Input: part model. Units: mm. Frame: model coordinates. A direction names the side the tool comes from. Coordinates: 2 decimals unless noted, no trailing zeros. Order: outer loops, then holes, each group sorted by start corner. A loop starts at its lowest first (then second) coordinate and runs counter-clockwise, first axis right, second up. Notation, with made-up numbers: (64.25, 32.5) -> (118.25, 32.5) arc R29 ccw to (118.25, 54.5) -> close; hole circle Ø7 at (54.25, 6.25). An arc over 180 degrees is marked (long way). One line per question, with ' | ' between items.
```python
from build123d import *

# Parameters (mm, degrees)
BOX004_W               = 20
BOX004_H               = 20
BOX004_DEPTH           = 80
BOX003_W               = 20
BOX003_H               = 20
BOX003_DEPTH           = 80
BOX002_W               = 10
BOX002_H               = 25
BOX002_DEPTH           = 35
BOX002_PITCH_ANGLE     = -15
BOX001_W               = 10
BOX001_H               = 25
BOX001_DEPTH           = 35
BOX001_PITCH_ANGLE     = 15
BOX_W                  = 20
BOX_H                  = 25
BOX_DEPTH              = 35
CYLINDER005_R          = 10
CYLINDER005_DEPTH      = 180
CYLINDER005_ROLL_ANGLE = 90
CYLINDER004_R          = 54
CYLINDER004_DEPTH      = 100
CYLINDER003_R          = 59
CYLINDER003_DEPTH      = 10
CYLINDER002_R          = 64
CYLINDER002_DEPTH      = 85
CYLINDER001_R          = 70
CYLINDER001_DEPTH      = 90
CYLINDER_R             = 77.5
CYLINDER_DEPTH         = 10
FILLET_R               = 3
FILLET001_R            = 5
FILLET002_R            = 5


with BuildPart() as tab_cut_l:
    # Box004 → Box004 (new body)
    with BuildSketch(Plane(origin=(-83, -10, 20), x_dir=(1, 0, 0), z_dir=(0, 0, 1))):
        with Locations((10, 10)):
            Rectangle(BOX004_W, BOX004_H)
    extrude(amount=BOX004_DEPTH)


with BuildPart() as tab_cut_r:
    # Box003 → Box003 (new body)
    with BuildSketch(Plane(origin=(63, -10, 20), x_dir=(1, 0, 0), z_dir=(0, 0, 1))):
        with Locations((10, 10)):
            Rectangle(BOX003_W, BOX003_H)
    extrude(amount=BOX003_DEPTH)


with BuildPart() as cube001:
    # Box002 → Box002 (new body)
    with BuildSketch(Plane.XY):
        with Locations((5, 12.5)):
            Rectangle(BOX002_W, BOX002_H)
    extrude(amount=BOX002_DEPTH)


with BuildPart() as cube001_1:
    # Box002 pitch: moved
    add(cube001.part.rotate(Axis((0, 0, 0), (0, 1, 0)), BOX002_PITCH_ANGLE))


with BuildPart() as cube001_2:
    # Box002 placement: moved
    add(cube001_1.part.moved(Location((-9.95, 48, 64))))


with BuildPart() as cube:
    # Box001 → Box001 (new body)
    with BuildSketch(Plane.XY):
        with Locations((5, 12.5)):
            Rectangle(BOX001_W, BOX001_H)
    extrude(amount=BOX001_DEPTH)


with BuildPart() as cube_1:
    # Box001 pitch: moved
    add(cube.part.rotate(Axis((0, 0, 0), (0, 1, 0)), BOX001_PITCH_ANGLE))


with BuildPart() as cube_2:
    # Box001 placement: moved
    add(cube_1.part.moved(Location((0, 48, 65))))


with BuildPart() as bearing_slot:
    # Box → Box (new body)
    with BuildSketch(Plane(origin=(-10, 48, 65), x_dir=(1, 0, 0), z_dir=(0, 0, 1))):
        with Locations((10, 12.5)):
            Rectangle(BOX_W, BOX_H)
    extrude(amount=BOX_DEPTH)


with BuildPart() as bearing_holes:
    # Cylinder005 → Cylinder005 (new body)
    with BuildSketch(Plane.XY):
        Circle(CYLINDER005_R)
    extrude(amount=CYLINDER005_DEPTH)


with BuildPart() as bearing_holes_1:
    # Cylinder005 roll: moved
    add(bearing_holes.part.rotate(Axis((0, 0, 0), (1, 0, 0)), CYLINDER005_ROLL_ANGLE))


with BuildPart() as bearing_holes_2:
    # Cylinder005 placement: moved
    add(bearing_holes_1.part.moved(Location((0, 90, 65))))


with BuildPart() as through_hole:
    # Cylinder004 → Cylinder004 (new body)
    with BuildSketch(Plane.XY):
        Circle(CYLINDER004_R)
    extrude(amount=CYLINDER004_DEPTH)


with BuildPart() as inner_lip:
    # Cylinder003 → Cylinder003 (new body)
    with BuildSketch(Plane.XY.offset(80)):
        Circle(CYLINDER003_R)
    extrude(amount=CYLINDER003_DEPTH)


with BuildPart() as inner_hole:
    # Cylinder002 → Cylinder002 (new body)
    with BuildSketch(Plane.XY):
        Circle(CYLINDER002_R)
    extrude(amount=CYLINDER002_DEPTH)


with BuildPart() as body_cylinder:
    # Cylinder001 → Cylinder001 (new body)
    with BuildSketch(Plane.XY.offset(5)):
        Circle(CYLINDER001_R)
    extrude(amount=CYLINDER001_DEPTH)


with BuildPart() as cut007:
    # Cylinder → Cylinder (new body)
    with BuildSketch(Plane.XY):
        Circle(CYLINDER_R)
    extrude(amount=CYLINDER_DEPTH)

    # Fusion: union Body_Cylinder
    add(body_cylinder.part)

    # Cut: cut Inner_Hole
    add(inner_hole.part, mode=Mode.SUBTRACT)

    # Fusion001: union Inner_Lip
    add(inner_lip.part)

    # Cut001: cut Through_Hole
    add(through_hole.part, mode=Mode.SUBTRACT)

    # Fillet
    fillet_edges = [cut007.edges().sort_by_distance(p)[0] for p in [
        (-70, 0, 10),
    ]]
    fillet(fillet_edges, radius=FILLET_R)

    # Fillet001
    fillet001_edges = [cut007.edges().sort_by_distance(p)[0] for p in [
        (-77.5, 0, 0),
    ]]
    fillet(fillet001_edges, radius=FILLET001_R)

    # Fillet002
    fillet002_edges = [cut007.edges().sort_by_distance(p)[0] for p in [
        (-70, 0, 95),
    ]]
    fillet(fillet002_edges, radius=FILLET002_R)

    # Cut002: cut Bearing_Holes
    add(bearing_holes_2.part, mode=Mode.SUBTRACT)

    # Cut003: cut Bearing_Slot
    add(bearing_slot.part, mode=Mode.SUBTRACT)

    # Cut004: cut Cube
    add(cube_2.part, mode=Mode.SUBTRACT)

    # Cut005: cut Cube001
    add(cube001_2.part, mode=Mode.SUBTRACT)

    # Cut006: cut Tab_Cut_R
    add(tab_cut_r.part, mode=Mode.SUBTRACT)

    # Cut007: cut Tab_Cut_L
    add(tab_cut_l.part, mode=Mode.SUBTRACT)


solid = cut007.part
```
1. Pin query (flat end, axial travel): pin 1 Ø1 at (y, z) = (-48, 19.5) entering from +X; pin 2 Ø1 at (x, z) = (41.5, 11.5) entering from -Y; pin 3 Ø10 at (y, z) = (-30, 80) entering from -X. Return the tip coordinate at first contact, or that it passes through.
Recorded:
pin 1: stops at x = 51.42 | pin 2: stops at y = -57.43 | pin 3: stops at x = -65.38
2. Cut plane C-C, the plane y = 0. Return loops of the section in (x, z), and give its area (3 significant figures).
Recorded:
outline: (-77.5, 5) arc R5 ccw to (-72.5, 0) -> (-64, 0) -> (-64, 20) -> (-70, 20) -> (-70, 13) arc R3 cw to (-73, 10) -> (-77.5, 10) -> close; (-63, 85) -> (-59, 85) -> (-59, 80) -> (-54, 80) -> (-54, 95) -> (-63, 95) -> close; (54, 80) -> (59, 80) -> (59, 85) -> (63, 85) -> (63, 95) -> (54, 95) -> close; (64, 0) -> (72.5, 0) arc R5 ccw to (77.5, 5) -> (77.5, 10) -> (73, 10) arc R3 cw to (70, 13) -> (70, 20) -> (64, 20) -> close | area: 613 mm^2
3. Cut plane A-A, the plane z = 43. Return loops of the section in (x, y).
Recorded:
outline: (-69.28, -10) arc R70 ccw to (69.28, -10) -> (63.21, -10) arc R64 cw to (-63.21, -10) -> close; (-69.28, 10) -> (-63.21, 10) arc R64 cw to (63.21, 10) -> (69.28, 10) arc R70 ccw to start
4. Cut plane B-B, the plane x = 0. Return loops of the section in (y, z), and give its area (3 significant figures).
Recorded:
outline: (-77.5, 5) arc R5 ccw to (-72.5, 0) -> (-64, 0) -> (-64, 55) -> (-70, 55) -> (-70, 13) arc R3 cw to (-73, 10) -> (-77.5, 10) -> close; (-70, 75) -> (-64, 75) -> (-64, 85) -> (-59, 85) -> (-59, 80) -> (-54, 80) -> (-54, 95) -> (-65, 95) arc R5 ccw to (-70, 90) -> close; (64, 0) -> (72.5, 0) arc R5 ccw to (77.5, 5) -> (77.5, 10) -> (73, 10) arc R3 cw to (70, 13) -> (70, 55) -> (64, 55) -> close | area: 1,040 mm^2
5. Ray query, line 1 (X direction, y = 0, z = 90); line 2 (X direction, y = -47, z = 84); line 3 (Y direction, x = 40, z = 61). Return the intervals inside material, ascending. Write a range as [from, to].
Recorded:
line 1: x = [-63, -54], [54, 63] | line 2: x = [-51.87, -43.44], [-35.67, -26.59], [26.59, 35.67], [43.44, 51.87] | line 3: y = [-57.45, -49.96], [49.96, 57.45]
6. Mould query, pull axis X, two halves, no side actions, for faces 1 (the face through (-2.242, -53.953, 87.395)), 2 (the face through (64.662, -26.81, 50.961)), 3 (the face through (-67, 0, 20)). Classes: released by +X, released by -X, zero draft, split by the parting line, or undercut.
Recorded:
face 1: undercut | face 2: split by the parting line | face 3: zero draft
7. Access query for faces 4 (the face through (63, 0, 90)), 5 (the face through (-28.4, -52, 85)), 6 (the face through (57, -46, 10)). Directions: +Z, -Z, +X, -X, +Y, -Y. A direction counts if a zero-diameter tool reaches every point of the face in a straight line with its end or side. Return the directions, or none.
Recorded:
face 4: +Z, -Z, +X | face 5: -Z | face 6: +Z
